Here's how the part is built. I have some questions about the finished solid (model axes, mm). A direction names the side the tool comes from. Give positions to 0.01 mm unless a question says otherwise; leave off trailing zeros. Loops run counter-clockwise (first coordinate to the right, second up) from the corner with the lowest first, then second, coordinate; pieces in that order, holes last. Notation, with made-up numbers: (-2.5, 72.25) -> (10.5, 72.25) arc R16 ccw to (10.5, 92.25) -> close; hole circle Ø4 at (-8.75, 57.5). An arc over 180 degrees is marked (long way). Answer in a Markdown table with one row per item. Add a question column.
Item 1: If we section it at A-A (x = 72.5): Write out the boundary of the cut face in (y, z), then the cut area to 3 significant figures.
Item 2: For P1, Ø10, axis at y = -7, z = 16, coming from the +X side; P2, Ø8, axis at x = -5, z = 21.5, coming from the +Y side; P3, Ø1.6, axis at x = 5.5, z = 46, coming from the +Y side (3 decimals); P4, Ø3, axis at x = 77.02, y = 0, coming from the -Z side, each with a flat end and sliding along its axis, tell me the tip position at first contact or that it passes through.
Item 3: If we section it at D-D (x = 31): Write out the boundary of the cut face in (y, z), then the cut area to 3 significant figures.
Item 4: If I drill on line 1 (X direction, y = 9, z = 29.5); line 2 (Z direction, x = 52.5, y = -11.5); line 3 (Y direction, x = 1, z = 44), over which ranges is the centre line in solid material (lowest first)?
Item 5: If we section it at B-B (z = 43): Write out the boundary of the cut face in (x, y) (3 decimals).
Item 6: Which directions (+Z, -Z, +X, -X, +Y, -Y) give clear straight access to the entire face, cutting with the end or side of a thin tool? Please do faces 1 (the face through (-42.413, 17.933, 6.451)), 2 (the face through (5, 5, 39.5)), 3 (the face through (0, -5, 45)), 4 (the face through (0, 5, 45)), 5 (the face through (-24.6, 0.56, 3.45)).
Item 7: We'd pull the mould along X, two halves only. Please class faces 6 (the face through (0.636, 44.996, 3.451)), 7 (the face through (-1, -18, 0)), 8 (the face through (-26.726, -1.559, 6.451)): released by +X, released by -X, zero draft, split by the parting line, or undercut.
Item 8: If we section it at C-C (y = 37): Write out the boundary of the cut face in (x, z), then the cut area to 3 significant figures.
```python
from build123d import *

# Parameters (mm, degrees)
ESQUISSE1_R                  = 85
ESQUISSE1_R_2                = 7.5
ESQUISSE1_R_3                = 4.5
BOSS_EXTRU_1_DEPTH           = 3
BOSS_EXTRU_2_DEPTH           = 4
BOSS_EXTRU_3_DEPTH           = 3
ESQUISSE5_R                  = 7.5
ENL_V_MAT_EXTRU_2_DEPTH      = 3
ENL_V_START                  = -3
ENL_V_MAT_EXTRU_3_DEPTH      = 3
ENL_V_MAT_EXTRU_6_DEPTH      = 2
ESQUISSE9_R                  = 17
ENL_V_MAT_EXTRU_4_DEPTH      = 0.25
ENL_V_MAT_EXTRU_5_DEPTH      = 10
ENL_V_MAT_EXTRU_5_DEPTH_BACK = 7.5
ESQUISSE10_OUTSIDE_W         = 220.994
ESQUISSE10_OUTSIDE_H         = 220.994
ESQUISSE10_OUTSIDE_R         = 6.75
ESQUISSE11_R                 = 1.45
BOSS_EXTRU_4_DEPTH           = 4
D_GAGEMENT_M31_D             = 3.4


with BuildPart() as part:
    # Esquisse1 → Boss.-Extru.1 (new body)
    with BuildSketch(Plane.XY):
        Circle(ESQUISSE1_R)
        Circle(ESQUISSE1_R_2, mode=Mode.SUBTRACT)
        with Locations((-72.5, -16)):
            Circle(ESQUISSE1_R_3, mode=Mode.SUBTRACT)
        with Locations((72.5, -16)):
            Circle(ESQUISSE1_R_3, mode=Mode.SUBTRACT)
    extrude(amount=BOSS_EXTRU_1_DEPTH)

    # Esquisse3 → Boss.-Extru.2 (add)
    with BuildSketch(Plane.XY.offset(3)):
        with BuildLine():
            Line((14.142135624, -14.142135624), (38.961482916, 10.677211668))
            ThreePointArc((38.961482916, 10.677211668), (42.400953744, 17.820746084), (40.634935389, 25.549990723))
            ThreePointArc((40.634935389, 25.549990723), (0, 48), (-40.634935389, 25.549990723))
            ThreePointArc((-40.634935389, 25.549990723), (-42.400953744, 17.820746084), (-38.961482916, 10.677211668))
            Line((-38.961482916, 10.677211668), (-14.142135624, -14.142135624))
            ThreePointArc((-14.142135624, -14.142135624), (0, -20), (14.142135624, -14.142135624))
        make_face()
        with BuildLine():
            Line((-36.840162572, 12.798532012), (-12.02081528, -12.02081528))
            ThreePointArc((-12.02081528, -12.02081528), (0, -17), (12.02081528, -12.02081528))
            Line((12.02081528, -12.02081528), (36.840162572, 12.798532012))
            ThreePointArc((36.840162572, 12.798532012), (39.419765694, 18.156182824), (38.095251927, 23.953116303))
            ThreePointArc((38.095251927, 23.953116303), (0, 45), (-38.095251927, 23.953116303))
            ThreePointArc((-38.095251927, 23.953116303), (-39.419765694, 18.156182824), (-36.840162572, 12.798532012))
        make_face(mode=Mode.SUBTRACT)
    extrude(amount=BOSS_EXTRU_2_DEPTH)

    # Esquisse4 → Boss.-Extru.3 (add)
    with BuildSketch(Plane.XY.offset(7)):
        with BuildLine():
            Line((-38.961482916, 10.677211668), (-14.142135624, -14.142135624))
            ThreePointArc((-14.142135624, -14.142135624), (0, -20), (14.142135624, -14.142135624))
            Line((14.142135624, -14.142135624), (38.961482916, 10.677211668))
            ThreePointArc((38.961482916, 10.677211668), (42.400953744, 17.820746084), (40.634935389, 25.549990723))
            ThreePointArc((40.634935389, 25.549990723), (0, 48), (-40.634935389, 25.549990723))
            ThreePointArc((-40.634935389, 25.549990723), (-42.400953744, 17.820746084), (-38.961482916, 10.677211668))
        make_face()
    extrude(amount=BOSS_EXTRU_3_DEPTH)

    # Esquisse5 → Enl_v. mat.-Extru.2 (cut)
    with BuildSketch(Plane(origin=(0, 0, 7), x_dir=(-1, 0, 0), z_dir=(0, 0, -1))):
        with Locations(Location((0, 0, 0), (0, 0, 180))):
            Circle(ESQUISSE5_R)
    extrude(amount=-ENL_V_MAT_EXTRU_2_DEPTH, mode=Mode.SUBTRACT)

    # Esquisse6 → Enl_v. mat.-Extru.3 (cut)
    with BuildSketch(Plane.XY.offset(3).offset(ENL_V_START)):
        with BuildLine():
            Line((-36.840162572, 12.798532012), (-12.02081528, -12.02081528))
            ThreePointArc((-12.02081528, -12.02081528), (0, -17), (12.02081528, -12.02081528))
            Line((12.02081528, -12.02081528), (36.840162572, 12.798532012))
            ThreePointArc((36.840162572, 12.798532012), (39.419765694, 18.156182824), (38.095251927, 23.953116303))
            ThreePointArc((38.095251927, 23.953116303), (0, 45), (-38.095251927, 23.953116303))
            ThreePointArc((-38.095251927, 23.953116303), (-39.419765694, 18.156182824), (-36.840162572, 12.798532012))
        make_face()
    extrude(amount=ENL_V_MAT_EXTRU_3_DEPTH, mode=Mode.SUBTRACT)

    # Esquisse7 → R_volution1 (revolve)
    with BuildSketch(Plane(origin=(0, 0, 0), x_dir=(0, 0, -1), z_dir=(1, 0, 0)), mode=Mode.PRIVATE) as r_volution1_sk:
        Polygon((-7, -7.5), (-38.5, -5.12), (-38.5, -4.12), (-47, -4.12), (-47, -11), (-7, -11), align=None)
    revolve(r_volution1_sk.sketch.rotate(Axis((0, 0, 0), (0, 0, 1)), 270), axis=Axis((0, 0, 0), (0, 0, 1)))

    # Esquisse8 → Enl_v. mat.-Extru.6 (cut)
    with BuildSketch(Plane.XY.offset(47)):
        with BuildLine():
            Line((3.293747865, 2.475), (10.717946398, 2.475))
            ThreePointArc((10.717946398, 2.475), (0, 11), (-10.717946398, 2.475))
            Line((-10.717946398, 2.475), (-3.293747865, 2.475))
            ThreePointArc((-3.293747865, 2.475), (0, 4.12), (3.293747865, 2.475))
        make_face()
        with BuildLine():
            Line((-10.717946398, -2.475), (-3.293747865, -2.475))
            ThreePointArc((-3.293747865, -2.475), (0, -4.12), (3.293747865, -2.475))
            Line((3.293747865, -2.475), (10.717946398, -2.475))
            ThreePointArc((10.717946398, -2.475), (0, -11), (-10.717946398, -2.475))
        make_face()
    extrude(amount=-ENL_V_MAT_EXTRU_6_DEPTH, mode=Mode.SUBTRACT)

    # Esquisse9 → Enl_v. mat.-Extru.4 (cut)
    with BuildSketch(Plane(origin=(0, 0, 7), x_dir=(-1, 0, 0), z_dir=(0, 0, -1))):
        Circle(ESQUISSE9_R)
    extrude(amount=-ENL_V_MAT_EXTRU_4_DEPTH, mode=Mode.SUBTRACT)

    # Esquisse10 outside → Enl_v. mat.-Extru.5 (cut, two sides: drawn at the far end of the back side and taken through both)
    with BuildSketch(Plane.XY.offset(47).offset(-ENL_V_MAT_EXTRU_5_DEPTH_BACK)):
        Rectangle(ESQUISSE10_OUTSIDE_W, ESQUISSE10_OUTSIDE_H)
        with Locations(Location((0, 0, 0), (0, 0, 201.510188267))):
            Circle(ESQUISSE10_OUTSIDE_R, mode=Mode.SUBTRACT)
    extrude(amount=ENL_V_MAT_EXTRU_5_DEPTH + ENL_V_MAT_EXTRU_5_DEPTH_BACK, mode=Mode.SUBTRACT)

    # Esquisse11 → Boss.-Extru.4 (add)
    with BuildSketch(Plane.XY.offset(10)):
        with Locations((0, 31.05)):
            Circle(ESQUISSE11_R)
    extrude(amount=BOSS_EXTRU_4_DEPTH)

    # D_gagement M31 (through all)
    with Locations(Plane.XY.offset(3)):
        with Locations((60.78495979, 42), (77.019852204, 0), (61.519852204, -42), (-60.78495979, -42), (-77.019852204, 0), (-61.519852204, 42)):
            Hole(D_GAGEMENT_M31_D / 2)


solid = part.part
```
Recorded:
| question | item | result |
|---|---|---|
| 1 | outline | (-44.37, 0) -> (-20.5, 0) -> (-20.5, 3) -> (-44.37, 3) -> close; (-11.5, 0) -> (44.37, 0) -> (44.37, 3) -> (-11.5, 3) -> close |
| 1 | area | 239 mm^2 |
| 2 | P1 | stops at x = 10.82 |
| 2 | P2 | stops at y = 10.95 |
| 2 | P3 | stops at y = 2.475 |
| 2 | P4 | passes through |
| 3 | outline | (-79.15, 0) -> (6.96, 0) -> (6.96, 7) -> (32.62, 7) -> (32.62, 0) -> (79.15, 0) -> (79.15, 3) -> (36.65, 3) -> (36.65, 10) -> (2.72, 10) -> (2.72, 3) -> (-79.15, 3) -> close |
| 3 | area | 533 mm^2 |
| 4 | line 1 | x = -6.32 to 6.32 |
| 4 | line 2 | z = 0 to 3 |
| 4 | line 3 | y = -6.68 to -4, 4 to 6.68 |
| 5 | outline | circle Ø13.5 at (0, 0); hole circle Ø8.24 at (0, 0) |
| 6 | face 1 | +Z, -X |
| 6 | face 2 | +Z |
| 6 | face 3 | +Z, +X, -X, -Y |
| 6 | face 4 | +Z, +X, -X, +Y |
| 6 | face 5 | -Z |
| 7 | face 6 | undercut |
| 7 | face 7 | zero draft |
| 7 | face 8 | released by -X |
| 8 | outline | (-76.52, 0) -> (-25.61, 0) -> (-25.61, 7) -> (25.61, 7) -> (25.61, 0) -> (76.52, 0) -> (76.52, 3) -> (30.58, 3) -> (30.58, 10) -> (-30.58, 10) -> (-30.58, 3) -> (-76.52, 3) -> close |
| 8 | area | 529 mm^2 |
